from build123d import *

# Parameters (mm, degrees)
SKETCH_1_R          = 1.75
EXTRUDE_1_DEPTH     = 6.6
EXTRUDE_1_2_DEPTH   = 6.6
SKETCH_2_R          = 50
EXTRUDE_2_DEPTH     = 3.4
SKETCH_4_R          = 1.75
CUT_EXTRUDE_2_DEPTH = 10
EXTRUDE_7_DEPTH     = 20
SKETCH_10_W         = 36
SKETCH_10_H         = 48.823085464
CUT_EXTRUDE_3_DEPTH = 10
SKETCH_11_R         = 3
CUT_EXTRUDE_6_DEPTH = 10


with BuildPart() as part:
    # Sketch 1 → Extrude 1 (new body)
    with BuildSketch(Plane.XY):
        with BuildLine():
            ThreePointArc((20.506096654, 20.506096654), (29, 0), (20.506096654, -20.506096654))
            Line((20.506096654, -20.506096654), (24.748737342, -24.748737342))
            ThreePointArc((24.748737342, -24.748737342), (24.748737342, -35.355339059), (35.355339059, -35.355339059))
            ThreePointArc((35.355339059, -35.355339059), (50, 0), (35.355339059, 35.355339059))
            ThreePointArc((35.355339059, 35.355339059), (24.748737342, 35.355339059), (24.748737342, 24.748737342))
            Line((24.748737342, 24.748737342), (20.506096654, 20.506096654))
        make_face()
        with Locations((30.0520382, 30.0520382)):
            Circle(SKETCH_1_R, mode=Mode.SUBTRACT)
        with Locations((30.0520382, -30.0520382)):
            Circle(SKETCH_1_R, mode=Mode.SUBTRACT)
        with Locations((42.5, 0)):
            Circle(SKETCH_1_R, mode=Mode.SUBTRACT)
    extrude(amount=EXTRUDE_1_DEPTH)



with BuildPart() as body_2:
    # Sketch 1 → Extrude 1 2 (new body)
    with BuildSketch(Plane.XY):
        with BuildLine():
            ThreePointArc((-35.355339059, 35.355339059), (-50, 0), (-35.355339059, -35.355339059))
            ThreePointArc((-35.355339059, -35.355339059), (-24.748737342, -35.355339059), (-24.748737342, -24.748737342))
            Line((-24.748737342, -24.748737342), (-20.506096654, -20.506096654))
            ThreePointArc((-20.506096654, -20.506096654), (-29, 0), (-20.506096654, 20.506096654))
            Line((-20.506096654, 20.506096654), (-24.748737342, 24.748737342))
            ThreePointArc((-24.748737342, 24.748737342), (-24.748737342, 35.355339059), (-35.355339059, 35.355339059))
        make_face()
        with Locations((-30.0520382, 30.0520382)):
            Circle(SKETCH_1_R, mode=Mode.SUBTRACT)
        with Locations((-30.0520382, -30.0520382)):
            Circle(SKETCH_1_R, mode=Mode.SUBTRACT)
        with Locations((-42.5, 0)):
            Circle(SKETCH_1_R, mode=Mode.SUBTRACT)
    extrude(amount=EXTRUDE_1_2_DEPTH)


with BuildPart() as part_1:
    add(part.part)

    add(body_2.part)  # Extrude 2 merges body 2
    # Sketch 2 → Extrude 2 (add)
    with BuildSketch(Plane.XY.offset(6.6)):
        with Locations(Location((0, 0, 0), (0, 0, 225))):
            Circle(SKETCH_2_R)
    extrude(amount=EXTRUDE_2_DEPTH)

    # Sketch 4 → Cut-Extrude 2 (cut, symmetric)
    with BuildSketch(Plane(origin=(0, 0, 6.6), x_dir=(-1, 0, 0), z_dir=(0, 0, -1))):
        with Locations(Location((-42.5, 0, 0), (0, 0, 180))):
            Circle(SKETCH_4_R)
        with Locations(Location((-30.0520382, 30.0520382, 0), (0, 0, 180))):
            Circle(SKETCH_4_R)
        with Locations(Location((-30.0520382, -30.0520382, 0), (0, 0, 180))):
            Circle(SKETCH_4_R)
        with Locations(Location((30.0520382, -30.0520382, 0), (0, 0, 180))):
            Circle(SKETCH_4_R)
        with Locations(Location((42.5, 0, 0), (0, 0, 180))):
            Circle(SKETCH_4_R)
        with Locations(Location((30.0520382, 30.0520382, 0), (0, 0, 180))):
            Circle(SKETCH_4_R)
    extrude(amount=CUT_EXTRUDE_2_DEPTH, both=True, mode=Mode.SUBTRACT)

    # Sketch 5 → Extrude 7 (add)
    with BuildSketch(Plane.XY.offset(10)):
        Polygon((-18, -31.176914536), (-18, -80), (18, -80), (18, -31.176914536), (36, 0), (18, 31.176914536), (18, 80), (-18, 80), (-18, 31.176914536), (-36, 0), align=None)
    extrude(amount=EXTRUDE_7_DEPTH)

    # Sketch 10 → Cut-Extrude 3 (cut)
    with BuildSketch(Plane.XY.offset(30)):
        with Locations((0, -55.588457268)):
            Rectangle(SKETCH_10_W, SKETCH_10_H)
        with Locations((0, 55.588457268)):
            Rectangle(SKETCH_10_W, SKETCH_10_H)
    extrude(amount=-CUT_EXTRUDE_3_DEPTH, mode=Mode.SUBTRACT)

    # Sketch 11 → Cut-Extrude 6 (cut)
    with BuildSketch(Plane.XY.offset(20)):
        with Locations((0, 62)):
            Circle(SKETCH_11_R)
    cut_extrude_6 = extrude(amount=-CUT_EXTRUDE_6_DEPTH, mode=Mode.SUBTRACT)

    # Mirror 2: Cut-Extrude 6 across plane
    add(cut_extrude_6.mirror(Plane.ZX), mode=Mode.SUBTRACT)


solid = part_1.part
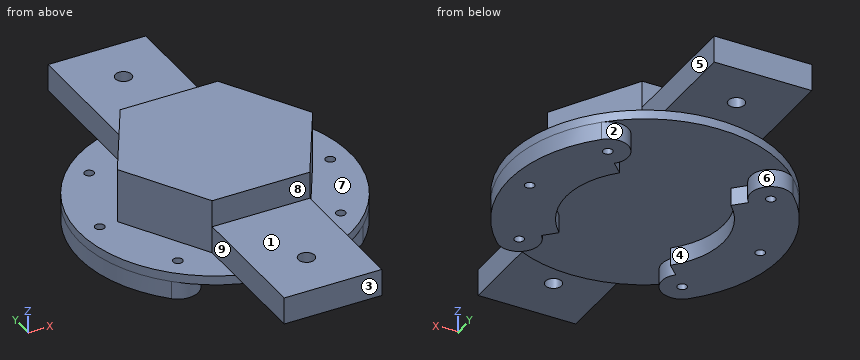
CAD build for the part. Positions are in the model's coordinates, mm. Face numbers are marked on the shaded views. A direction names the side the tool comes from. Round coordinates to 2 decimals unless told otherwise and drop trailing zeros. Write each loop counter-clockwise with the first axis right and the second up, starting at its lowest first coordinate (ties: lowest second). Pieces come first, ordered by that corner, then holes.
(1) Slice it at D-D, the plane z = 16.25. Write the cut outline in (x, y), and give its area (3 significant figures).
(2) Mould opens along Y. For the marked faces 1, 2, 3 and 4 say: pulls with the +Y half, pulls with the -Y half, needs draft (parallel to the pull), parting line crosses it, or undercut.
(3) Slice it at C-C, the plane y = -62. Write the cut outline in (x, z).
(4) Slice it at A-A, the plane x = 0. Write the cut outline in (y, z), and give its area (3 significant figures).
(5) Slice it at B-B, the plane z = 4.75. Write the cut outline in (x, y), and give its area (3 significant figures).
(6) 3-axis set-ups, long thin cutter, end or side, ignore diameter. For the marked faces 5, 6, 7, 8 and 9: which of +Z, -Z, +X, -X, +Y, -Y reach the whole face in a straight line?
(7) Drop flat-ended pins along their axis: P1, Ø1, axis at x = 38.5, y = 7, coming from the +Z side; P2, Ø11, axis at x = 8.5, y = 49.5, coming from the +Z side; P3, Ø1.5, axis at y = -10, z = 16, coming from the +X side; P4, Ø5.5, axis at x = 0, y = -62, coming from the -Z side. Give the stop position or say it passes through.
(8) Probe line 1 along Y through (x, z) = (0, 17.5); line 2 along X through (y, z) = (0, 4.5); line 3 along X through (y, z) = (-69, 12). List the from-to ranges inside material, lowest first.
From the geometry:
1. outline: (-36, 0) - (-18, -31.18) - (-18, -80) - (18, -80) - (18, -31.18) - (36, 0) - (18, 31.18) - (18, 80) - (-18, 80) - (-18, 31.18) - close; hole circle Ø6 at (0, -62); hole circle Ø6 at (0, 62)
1. area: 6,830 mm2
2. face 1: needs draft
2. face 2: undercut
2. face 3: pulls with the -Y half
2. face 4: undercut
3. outline: (-18, 10) - (-3, 10) - (-3, 20) - (-18, 20) - close; (3, 10) - (18, 10) - (18, 20) - (3, 20) - close
4. outline: (-80, 10) - (-65, 10) - (-65, 20) - (-80, 20) - close; (-59, 10) - (-50, 10) - (-50, 6.6) - (50, 6.6) - (50, 10) - (59, 10) - (59, 20) - (31.18, 20) - (31.18, 30) - (-31.18, 30) - (-31.18, 20) - (-59, 20) - close; (65, 10) - (80, 10) - (80, 20) - (65, 20) - close
4. area: 2,440 mm2
5. outline: (-35.36, -35.36) arc R7.5 ccw to (-24.75, -24.75) - (-20.51, -20.51) arc R29 cw to (-20.51, 20.51) - (-24.75, 24.75) arc R7.5 ccw to (-35.36, 35.36) arc R50 ccw to start; (20.51, -20.51) - (24.75, -24.75) arc R7.5 ccw to (35.36, -35.36) arc R50 ccw to (35.36, 35.36) arc R7.5 ccw to (24.75, 24.75) - (20.51, 20.51) arc R29 cw to start; hole circle Ø3.5 at (-42.5, 0); hole circle Ø3.5 at (-30.05, -30.05); hole circle Ø3.5 at (-30.05, 30.05); hole circle Ø3.5 at (30.05, -30.05); hole circle Ø3.5 at (30.05, 30.05); hole circle Ø3.5 at (42.5, 0)
5. area: 2,900 mm2
6. face 5: +Z, +X, +Y
6. face 6: -Z
6. face 7: +Z, +X
6. face 8: +Z, +X, -X, -Y
6. face 9: +Z, -X, -Y
7. P1: stops at z = 10
7. P2: stops at z = 20
7. P3: stops at x = 30.66
7. P4: passes through
8. line 1: y = -80 to -65, -59 to 59, 65 to 80
8. line 2: x = -50 to -44.25, -40.75 to -29, 29 to 40.75, 44.25 to 50
8. line 3: x = -18 to 18
